The model under review builds one solid part; all positions refer to its coordinate system, in mm. Round coordinates to 2 decimals unless told otherwise and drop trailing zeros. Order: outer loops, then holes, each group sorted by start corner. A loop starts at its lowest first (then second) coordinate and runs counter-clockwise, first axis right, second up. Notation, with made-up numbers: (12.5, 74) -> (62.5, 74) arc R22 ccw to (62.5, 97) -> close; hole circle Ø8 at (-25, -25.75). An arc over 180 degrees is marked (long way). Return JSON: item names as keys, results as strings. Group by question number.
from build123d import *

# Parameters (mm, degrees)
SKETCH1_R           = 2
SKETCH1_R_2         = 3
BOSS_EXTRUDE1_DEPTH = 4.7625
SKETCH4_W           = 20
SKETCH4_H           = 20
CUT_EXTRUDE2_DEPTH  = 0.01


with BuildPart() as part:
    # Sketch1 → Boss-Extrude1 (new body)
    with BuildSketch(Plane.XY):
        with BuildLine():
            Line((-14.25, -9.45), (-14.25, 13.336101268))
            ThreePointArc((-14.25, 13.336101268), (-13.704321085, 15.607449693), (-12.186390533, 17.383027341))
            ThreePointArc((-12.186390533, 17.383027341), (90, 50.55), (192.186390533, 17.383027341))
            ThreePointArc((192.186390533, 17.383027341), (193.704321085, 15.607449693), (194.25, 13.336101268))
            Line((194.25, 13.336101268), (194.25, -9.45))
            ThreePointArc((194.25, -9.45), (192.785533906, -12.985533906), (189.25, -14.45))
            Line((189.25, -14.45), (167.269740757, -14.45))
            ThreePointArc((167.269740757, -14.45), (165.828788887, -14.237865674), (164.510107159, -13.619463083))
            ThreePointArc((164.510107159, -13.619463083), (90, 8.80503367), (15.489892841, -13.619463083))
            ThreePointArc((15.489892841, -13.619463083), (14.171211113, -14.237865674), (12.730259243, -14.45))
            Line((12.730259243, -14.45), (-9.25, -14.45))
            ThreePointArc((-9.25, -14.45), (-12.785533906, -12.985533906), (-14.25, -9.45))
        make_face()
        with Locations((74, 43.4)):
            Circle(SKETCH1_R, mode=Mode.SUBTRACT)
        with Locations((74, 14.4)):
            Circle(SKETCH1_R, mode=Mode.SUBTRACT)
        with Locations((114, 43.4)):
            Circle(SKETCH1_R, mode=Mode.SUBTRACT)
        with Locations((114, 14.4)):
            Circle(SKETCH1_R, mode=Mode.SUBTRACT)
        with Locations((180, 0)):
            Circle(SKETCH1_R_2, mode=Mode.SUBTRACT)
        Circle(SKETCH1_R_2, mode=Mode.SUBTRACT)
        with Locations((4, 18.4)):
            Circle(SKETCH1_R_2, mode=Mode.SUBTRACT)
        with Locations((176, 18.4)):
            Circle(SKETCH1_R_2, mode=Mode.SUBTRACT)
    extrude(amount=BOSS_EXTRUDE1_DEPTH)

    # Sketch4 → Cut-Extrude2 (cut)
    with BuildSketch(Plane.XY):
        Rectangle(SKETCH4_W, SKETCH4_H)
        with Locations((180, 0)):
            Rectangle(SKETCH4_W, SKETCH4_H)
    extrude(amount=CUT_EXTRUDE2_DEPTH, mode=Mode.SUBTRACT)


solid = part.part
Item 1: The part is to be moulded in two halves that separate along Y. For faces 1 (the face through (182.86, 0.9, 2.35)), 2 (the face through (192.82, -12.95, 2.35)), 3 (the face through (177.6, 2.4, 0.01)), say which applies: +Y half, -Y half, draft (parallel to the pull), parting line (faces both ways), or undercut.
Item 2: Wall thickness on line 1 along Y through (x, z) = (74, 3.65); line 2 along X through (y, z) = (21, 1.85); line 3 along Y through (x, z) = (181, 2): over which ranges is each line inside the solid? List them lowest first.
Item 3: Consider section C-C on y = 43.4. State the section outline as (x, z) points, plus the area to 3 significant figures.
Item 4: Consider section D-D on x = 74. State the section outline as (y, z) points, plus the area to 3 significant figures.
Item 5: Insertion check: pin 1 Ø1 at (y, z) = (22, 1.5) entering from +X. The pin has a flat end and moves straight along its axis. Give the tip position at first contact, or say it passes through.
Item 6: Consider section A-A on z = 0.9. Give the number of separate pieces and of enclosed holes in the cut face, plus the area to 3 significant figures.
Values:
{
 "1": {"face 1": "undercut", "face 2": "-Y half", "face 3": "draft"},
 "2": {"line 1": "7.85 to 12.4, 16.4 to 41.4, 45.4 to 49.81", "line 2": "-7.01 to 2.5, 5.5 to 174.5, 177.5 to 187.01", "line 3": "-14.45 to -2.83, 2.83 to 24.86"},
 "3": {"outline": "(40.63, 0) -> (72, 0) -> (72, 4.76) -> (40.63, 4.76) -> close; (76, 0) -> (112, 0) -> (112, 4.76) -> (76, 4.76) -> close; (116, 0) -> (139.37, 0) -> (139.37, 4.76) -> (116, 4.76) -> close", "area": "432 mm^2"},
 "4": {"outline": "(7.85, 0) -> (12.4, 0) -> (12.4, 4.76) -> (7.85, 4.76) -> close; (16.4, 0) -> (41.4, 0) -> (41.4, 4.76) -> (16.4, 4.76) -> close; (45.4, 0) -> (49.81, 0) -> (49.81, 4.76) -> (45.4, 4.76) -> close", "area": "162 mm^2"},
 "5": {"pin 1": "x = 186.26"},
 "6": {"separate pieces": "1", "enclosed holes": "8", "area": "8,680 mm^2"}
}
